Read the model definition and answer for the solid it produces. Units are mm, in the model's axes. A direction names the side the tool comes from. Give positions to 0.01 mm unless a question says otherwise; leave off trailing zeros. Loops run counter-clockwise (first coordinate to the right, second up) from the corner with the lowest first, then second, coordinate; pieces in that order, holes last. Notation, with made-up numbers: (55, -8) - (74, -8) arc R12 cw to (74, 10) - close; hole circle Ø8 at (50.25, -11.75). An arc over 180 degrees is marked (long way). Put each result on its own line as item: value. Start each with the question number.
1. A cutting plane is placed at A-A, the plane y = 0. Determine the outline of the cut face in (x, z), plus the area to 3 significant figures.
2. Consider L1, parallel to Y at x = 0, z = 86; L2, parallel to Z at x = 8, y = -14; L3, parallel to Z at x = 21.5, y = 35. Determine where each line is inside the solid, lowest interval first. Write a range as from..to.
3. For faces 1 (the cylindrical face through (37.64, -15.61, 53.98)), 2 (the flat face through (0, 0, 148)), 3 (the cylindrical face through (-11.99, 0.53, 142.93)), determine the directions among +Z, -Z, +X, -X, +Y, -Y from which every point of the face is accessible in a straight line to the end or side of a thin tool.
4. A cutting plane is placed at D-D, the plane z = 116.5. Determine the outline of the cut face in (x, y).
5. Given pin 1 Ø4 at (y, z) = (9, 83) entering from -X; pin 2 Ø24.5 at (x, y) = (-2, 11.5) entering from -Z; pin 3 Ø8 at (y, z) = (13.5, 78.5) entering from +X, each flat-ended and moving along its own axis, determine where each tip first touches the part or whether it passes through.
6. A cutting plane is placed at C-C, the plane z = 52.5. Determine the outline of the cut face in (x, y), plus the area to 3 significant figures.
7. For a pull along Y with two mould halves and no side action, classify faces 4 (the flat face through (-7, 10, 138)), 5 (the flat face through (-1, 1, 109.5)), 6 (the cylindrical face through (-31.1, 28.6, 54.7)) as released by +Y, released by -Y, zero draft, split by the parting line, or undercut.
```python
from build123d import *

# Parameters (mm, degrees)
F0_R     = 42.25
F1_DEPTH = 111
F2_T     = -1.5
F3_R     = 15
F4_DEPTH = 27
F5_R     = 12
F6_DEPTH = 10


with BuildPart() as f1:
    # F0 (on Top) → F1 (new body)
    with BuildSketch(Plane.XY):
        Circle(F0_R)
    extrude(amount=F1_DEPTH)

    # F2
    f2_openings = [f1.faces().sort_by_distance(p)[0] for p in [
        (0, 0, 0),
    ]]
    offset(amount=F2_T, openings=f2_openings)

    # F3 (on face) → F4 (join)
    with BuildSketch(Plane.XY.offset(111)):
        Circle(F3_R)
    extrude(amount=F4_DEPTH)

    # F5 (on face) → F6 (join)
    with BuildSketch(Plane.XY.offset(138)):
        Circle(F5_R)
    extrude(amount=F6_DEPTH)


solid = f1.part
```
Return value:
1. outline: (-42.25, 0) - (-40.75, 0) - (-40.75, 109.5) - (40.75, 109.5) - (40.75, 0) - (42.25, 0) - (42.25, 111) - (15, 111) - (15, 138) - (12, 138) - (12, 148) - (-12, 148) - (-12, 138) - (-15, 138) - (-15, 111) - (-42.25, 111) - close
1. area: 1,510 mm2
2. L1: y = -42.25..-40.75, 40.75..42.25
2. L2: z = 109.5..111
2. L3: z = 0..111
3. face 1: -Z
3. face 2: +Z, +X, -X, +Y, -Y
3. face 3: +Z
4. outline: circle Ø30 at (0, 0)
5. pin 1: stops at x = -41.67
5. pin 2: stops at z = 109.5
5. pin 3: stops at x = 41.17
6. outline: circle Ø84.5 at (0, 0); hole circle Ø81.5 at (0, 0)
6. area: 391 mm2
7. face 4: zero draft
7. face 5: undercut
7. face 6: split by the parting line
